Source: CAD feature listing. Evaluate the final solid. Frame: model axes, mm. Give positions to 0.01 mm unless a question says otherwise; leave off trailing zeros. Order: outer loops, then holes, each group sorted by start corner. A loop starts at its lowest first (then second) coordinate and runs counter-clockwise, first axis right, second up.
```python
from build123d import *

# Parameters (mm, degrees)
SKICA2_R                = 2.5
SKICA2_W                = 4.5
SKICA2_H                = 6
SKICA2_W_2              = 3
SKICA2_H_2              = 13
SKICA2_W_3              = 14
SKICA2_H_3              = 3.2
P_IDAT_VYSUNUT_M1_DEPTH = 3
ZAOBLIT1_R              = 15


with BuildPart() as part:
    # Skica2 → Přidat vysunutím1 (new body)
    with BuildSketch(Plane.XY):
        with BuildLine():
            Line((-62.5, 7.5), (-61.3, 7.5))
            ThreePointArc((-61.3, 7.5), (-52.847781356, 11.3), (-44.395562713, 7.5))
            Line((-44.395562713, 7.5), (-44.395562713, 3))
            Line((-44.395562713, 3), (-41.953287334, 3))
            ThreePointArc((-41.953287334, 3), (-41.547781356, 0), (-41.953287334, -3))
            Line((-41.953287334, -3), (-44.395562713, -3))
            Line((-44.395562713, -3), (-44.395562713, -7.5))
            ThreePointArc((-44.395562713, -7.5), (-52.847781356, -11.3), (-61.3, -7.5))
            Line((-61.3, -7.5), (-62.5, -7.5))
            Line((-62.5, -7.5), (-62.5, -32.5))
            Line((-62.5, -32.5), (62.5, -32.5))
            Line((62.5, -32.5), (62.5, -7.5))
            Line((62.5, -7.5), (61.3, -7.5))
            ThreePointArc((61.3, -7.5), (52.847781356, -11.3), (44.395562713, -7.5))
            Line((44.395562713, -7.5), (44.395562713, -3))
            Line((44.395562713, -3), (41.953287334, -3))
            ThreePointArc((41.953287334, -3), (41.547781356, 0), (41.953287334, 3))
            Line((41.953287334, 3), (44.395562713, 3))
            Line((44.395562713, 3), (44.395562713, 7.5))
            ThreePointArc((44.395562713, 7.5), (52.847781356, 11.3), (61.3, 7.5))
            Line((61.3, 7.5), (62.5, 7.5))
            Line((62.5, 7.5), (62.5, 32.5))
            Line((62.5, 32.5), (-62.5, 32.5))
            Line((-62.5, 32.5), (-62.5, 7.5))
        make_face()
        with Locations((-36, 24)):
            Circle(SKICA2_R, mode=Mode.SUBTRACT)
        with Locations((36, 24)):
            Circle(SKICA2_R, mode=Mode.SUBTRACT)
        with Locations((-36, -24)):
            Circle(SKICA2_R, mode=Mode.SUBTRACT)
        with Locations((36, -24)):
            Circle(SKICA2_R, mode=Mode.SUBTRACT)
        with Locations((-36.297781356, 0)):
            Rectangle(SKICA2_W, SKICA2_H, mode=Mode.SUBTRACT)
        with Locations((-43.047781356, -20.7)):
            Rectangle(SKICA2_W_2, SKICA2_H_2, mode=Mode.SUBTRACT)
        with Locations((-43.047781356, 20.7)):
            Rectangle(SKICA2_W_2, SKICA2_H_2, mode=Mode.SUBTRACT)
        with Locations((43.047781356, -20.7)):
            Rectangle(SKICA2_W_2, SKICA2_H_2, mode=Mode.SUBTRACT)
        with Locations((43.047781356, 20.7)):
            Rectangle(SKICA2_W_2, SKICA2_H_2, mode=Mode.SUBTRACT)
        with Locations((36.297781356, 0)):
            Rectangle(SKICA2_W, SKICA2_H, mode=Mode.SUBTRACT)
        with Locations((-24, 18)):
            Rectangle(SKICA2_W_3, SKICA2_H_3, mode=Mode.SUBTRACT)
        with Locations((-24, 10.8)):
            Rectangle(SKICA2_W_3, SKICA2_H_3, mode=Mode.SUBTRACT)
        with Locations((-24, 3.6)):
            Rectangle(SKICA2_W_3, SKICA2_H_3, mode=Mode.SUBTRACT)
        with Locations((-24, -3.6)):
            Rectangle(SKICA2_W_3, SKICA2_H_3, mode=Mode.SUBTRACT)
        with Locations((-24, -10.8)):
            Rectangle(SKICA2_W_3, SKICA2_H_3, mode=Mode.SUBTRACT)
        with Locations((-24, -18)):
            Rectangle(SKICA2_W_3, SKICA2_H_3, mode=Mode.SUBTRACT)
        with Locations((24, -18)):
            Rectangle(SKICA2_W_3, SKICA2_H_3, mode=Mode.SUBTRACT)
        with Locations((24, -10.8)):
            Rectangle(SKICA2_W_3, SKICA2_H_3, mode=Mode.SUBTRACT)
        with Locations((24, -3.6)):
            Rectangle(SKICA2_W_3, SKICA2_H_3, mode=Mode.SUBTRACT)
        with Locations((24, 3.6)):
            Rectangle(SKICA2_W_3, SKICA2_H_3, mode=Mode.SUBTRACT)
        with Locations((24, 10.8)):
            Rectangle(SKICA2_W_3, SKICA2_H_3, mode=Mode.SUBTRACT)
        with Locations((24, 18)):
            Rectangle(SKICA2_W_3, SKICA2_H_3, mode=Mode.SUBTRACT)
    extrude(amount=P_IDAT_VYSUNUT_M1_DEPTH)

    # Zaoblit1
    zaoblit1_edges = [part.edges().sort_by_distance(p)[0] for p in [
        (-62.5, 32.5, 1.5),
        (62.5, 32.5, 1.5),
        (62.5, -32.5, 1.5),
        (-62.5, -32.5, 1.5),
    ]]
    fillet(zaoblit1_edges, radius=ZAOBLIT1_R)


solid = part.part
```
1) Section query B-B, the plane y = -24. Return the cut outline in (x, z), and give its area (3 significant figures).
Report:
outline: (-61.02, 0) - (-44.55, 0) - (-44.55, 3) - (-61.02, 3) - close; (-41.55, 0) - (-38.5, 0) - (-38.5, 3) - (-41.55, 3) - close; (-33.5, 0) - (33.5, 0) - (33.5, 3) - (-33.5, 3) - close; (38.5, 0) - (41.55, 0) - (41.55, 3) - (38.5, 3) - close; (44.55, 0) - (61.02, 0) - (61.02, 3) - (44.55, 3) - close
area: 318 mm2
2) Pin query (flat end, axial travel): pin 1 (1.5 mm diameter, centred on y = -3.5, z = 1.5, fed in from -X). Return the tip coordinate at first contact, or that it passes through.
Report:
pin 1: stops at x = -44.4
3) Material intervals for L1, parallel to Y at x = 36, z = 1.8; L2, parallel to X at y = 4, z = 2.4; L3, parallel to X at y = 11.5, z = 0.7, sorted ascending.
Report:
L1: y = -32.5 to -26.5, -21.5 to -3, 3 to 21.5, 26.5 to 32.5
L2: x = -44.4 to -31, -17 to 17, 31 to 44.4
L3: x = -62.5 to -31, -17 to 17, 31 to 62.5
4) Draft query along Y for faces 1 (the flat face through (24, -12.4, 1)), 2 (the flat face through (-1, 0, 0)), 3 (the cylindrical face through (57.99, 28.22, 1.52)). Return one class per face: +Y half, -Y half, draft (parallel to the pull), parting line (faces both ways), or undercut.
Report:
face 1: undercut
face 2: draft
face 3: +Y half
5) Section query C-C, the plane z = 0.55. Count the separate pieces of the cut face and the enclosed holes in it, and give its area (3 significant figures).
Report:
separate pieces: 1
enclosed holes: 22
area: 6,350 mm2
6) Section query A-A, the plane x = -36. Return the cut outline in (y, z).
Report:
outline: (-32.5, 0) - (-26.5, 0) - (-26.5, 3) - (-32.5, 3) - close; (-21.5, 0) - (-3, 0) - (-3, 3) - (-21.5, 3) - close; (3, 0) - (21.5, 0) - (21.5, 3) - (3, 3) - close; (26.5, 0) - (32.5, 0) - (32.5, 3) - (26.5, 3) - close
